from build123d import *

# Parameters (mm, degrees)
BOSS_EXTRUDE1_DEPTH               = 36
BOSS_EXTRUDE2_DEPTH               = 8
FILLET1_R                         = 15
BOSS_EXTRUDE3_START               = 5
SKETCH3_R                         = 15
BOSS_EXTRUDE3_DEPTH               = 5
HOLE1_D                           = 12
HOLE1_DEPTH                       = 27.75
FILLET2_R                         = 12
M12X1_25_TAPPED_HOLE1_D           = 10.8
M12X1_25_TAPPED_HOLE1_DEPTH       = 24.505352657
M12X1_25_TAPPED_HOLE1_CSINK_D     = 12.05
M12X1_25_TAPPED_HOLE1_CSINK_ANGLE = 90
M12X1_25_TAPPED_HOLE1_TIP         = 3.244647343
RIB1_REACH                        = 92.255
SKETCH8_WALL_W                    = 228.161236354
SKETCH8_WALL_H                    = 10


with BuildPart() as part:
    # Sketch1 → Boss-Extrude1 (new, symmetric)
    with BuildSketch(Plane.XY):
        Polygon((0, 0), (0, 6), (5, 6), (5, 10), (35, 10), (35, 0), align=None)
    extrude(amount=BOSS_EXTRUDE1_DEPTH, both=True)

    # Sketch2 → Boss-Extrude2 (add)
    with BuildSketch(Plane.ZY.offset(-5)):
        with BuildLine():
            Line((-15, 60), (-15, 10))
            Line((-15, 10), (15, 10))
            Line((15, 10), (15, 60))
            ThreePointArc((15, 60), (0, 75), (-15, 60))
        make_face()
    extrude(amount=-BOSS_EXTRUDE2_DEPTH)

    # Fillet1
    fillet1_edges = [part.edges().sort_by_distance(p)[0] for p in [
        (9, 10, 15),
        (9, 10, -15),
    ]]
    fillet(fillet1_edges, radius=FILLET1_R)

    # Sketch3 → Boss-Extrude3 (add)
    with BuildSketch(Plane.ZY.offset(-5).offset(BOSS_EXTRUDE3_START)):
        with Locations((0, 60)):
            Circle(SKETCH3_R)
    extrude(amount=-BOSS_EXTRUDE3_DEPTH)

    # Hole1
    with Locations(Plane(origin=(13, 0, 0), x_dir=(0, 0, -1), z_dir=(1, 0, 0))):
        with Locations((0, 60)):
            Hole(HOLE1_D / 2, depth=HOLE1_DEPTH)

    # Fillet2
    fillet2_edges = [part.edges().sort_by_distance(p)[0] for p in [
        (35, 5, -36),
        (35, 5, 36),
    ]]
    fillet(fillet2_edges, radius=FILLET2_R)

    # M12x1.25 Tapped Hole1
    with Locations(Plane(origin=(0, 10, 0), x_dir=(1, 0, 0), z_dir=(0, 1, 0))):
        with Locations((23, -24), (23, 24)):
            CounterSinkHole(M12X1_25_TAPPED_HOLE1_D / 2, M12X1_25_TAPPED_HOLE1_CSINK_D / 2, depth=M12X1_25_TAPPED_HOLE1_DEPTH, counter_sink_angle=M12X1_25_TAPPED_HOLE1_CSINK_ANGLE)
            with Locations((0, 0, -(M12X1_25_TAPPED_HOLE1_DEPTH + M12X1_25_TAPPED_HOLE1_TIP / 2))):  # 118° drill point
                Cone(0, M12X1_25_TAPPED_HOLE1_D / 2, M12X1_25_TAPPED_HOLE1_TIP, mode=Mode.SUBTRACT)

    # Sketch8 wall → Rib1 (add, up to next)
    with BuildSketch(Plane(origin=(24, 30, 0), x_dir=(-0.481918749772, 0.876215908677, 0), z_dir=(-0.876215908677, -0.481918749772, 0)), mode=Mode.PRIVATE) as rib1_sk1:
        Rectangle(SKETCH8_WALL_W, SKETCH8_WALL_H)
    rib1_tool1 = extrude(rib1_sk1.sketch, amount=RIB1_REACH, mode=Mode.PRIVATE) - part.part
    add(rib1_tool1.solids().sort_by_distance((24, 30, 0))[0])


solid = part.part
CAD build for the part. Positions are in the model's coordinates, mm. A direction names the side the tool comes from. Give positions to 0.01 mm unless a question says otherwise; leave off trailing zeros. Write each loop counter-clockwise with the first axis right and the second up, starting at its lowest first coordinate (ties: lowest second). Pieces come first, ordered by that corner, then holes. Notation, with made-up numbers: (-6.75, 79) -> (31.25, 79) arc R24 ccw to (31.25, 100) -> close; hole circle Ø9 at (38, 33). An arc over 180 degrees is marked (long way). Return JSON: item names as keys, results as strings.
Item 1: Band-saw the part on B-B (x = 11.5). List the corners of the cut face in (y, z), then the cut area to 3 significant figures.
Answer below:
{"outline": "(0, -36) -> (10, -36) -> (10, -30) arc R15 cw to (25, -15) -> (60, -15) arc R15 ccw to (60, 15) -> (25, 15) arc R15 cw to (10, 30) -> (10, 36) -> (0, 36) -> close; hole circle Ø12 at (60, 0)", "area": "2,560 mm2"}
Item 2: Tool access for faces 1 (the flat face through (23, 10, 17)), 2 (the flat face through (9, 42, 15)), 3 (the flat face through (9, 43, -15)), 4 (the flat face through (23, 10, -17)): list every direction of +Z, -Z, +X, -X, +Y, -Y with a clear straight run to the whole face (end or side of a thin tool).
Answer below:
{"face 1": "+Z, +X, +Y", "face 2": "+Z, +X, -X, +Y", "face 3": "-Z, +X, -X, +Y", "face 4": "-Z, +X, +Y"}
Item 3: Drill centre lines: probe 1 along Z at (x, y) = (23, 2.5); probe 2 along X at (y, z) = (2, 24); probe 3 along Z at (x, y) = (20.5, 6). Where is each one in solid material? Low to high.
Answer below:
{"probe 1": "z = -36 to -29.4, -18.6 to 18.6, 29.4 to 36", "probe 2": "x = 0 to 17.6, 28.4 to 35", "probe 3": "z = -36 to -28.79, -19.21 to 19.21, 28.79 to 36"}
Item 4: Band-saw the part on D-D (y = 61.5). List the corners of the cut face in (x, z), then the cut area to 3 significant figures.
Answer below:
{"outline": "(0, -14.92) -> (13, -14.92) -> (13, -5.81) -> (0, -5.81) -> close; (0, 5.81) -> (13, 5.81) -> (13, 14.92) -> (0, 14.92) -> close", "area": "237 mm2"}
Item 5: Drop flat-ended pins along their axis: pin 1 (1.5 mm diameter, centred on x = 3.5, z = -9.5, fed in from +Y); pin 2 (11 mm diameter, centred on x = 22.5, y = 23.5, fed in from -Z); pin 3 (10 mm diameter, centred on y = 33.5, z = -14.5, fed in from -X); pin 4 (6.5 mm diameter, centred on x = 23, z = -24, fed in from -Y). Give the stop position or say it passes through.
Answer below:
{"pin 1": "stops at y = 72.18", "pin 2": "stops at z = -5", "pin 3": "stops at x = 5", "pin 4": "passes through"}
Item 6: Two-plate mould, pull along Z, no slides. Class faces 5 (the cylindrical face through (17.85, 4.62, 22.38)), 6 (the flat face through (0, 60.2, 6.5)), 7 (the cylindrical face through (9.06, 14.28, -19.51)): +Z half, -Z half, draft (parallel to the pull), parting line (faces both ways), or undercut.
Answer below:
{"face 5": "undercut", "face 6": "draft", "face 7": "-Z half"}
Item 7: Band-saw the part on C-C (y = 44). List the corners of the cut face in (x, z), then the cut area to 3 significant figures.
Answer below:
{"outline": "(5, -15) -> (13, -15) -> (13, -5) -> (16.3, -5) -> (16.3, 5) -> (13, 5) -> (13, 15) -> (5, 15) -> close", "area": "273 mm2"}
Item 8: Band-saw the part on A-A (z = 0). List the corners of the cut face in (x, y).
Answer below:
{"outline": "(0, 0) -> (35, 0) -> (35, 10) -> (13, 50) -> (13, 54) -> (0, 54) -> (0, 45) -> (5, 45) -> (5, 6) -> (0, 6) -> close; (0, 66) -> (13, 66) -> (13, 75) -> (0, 75) -> close"}
